Source: CAD feature listing. Evaluate the final solid. Frame: model axes, mm. A direction names the side the tool comes from. Round coordinates to 2 decimals unless told otherwise and drop trailing zeros. Loops run counter-clockwise (first coordinate to the right, second up) from the corner with the lowest first, then second, coordinate; pieces in that order, holes last. Notation, with made-up numbers: (32, 40) - (71, 40) arc R20 cw to (71, 55) - close; hole circle Ø6 at (-14, 39.25). An arc over 180 degrees is marked (long way). One line per question, with ' | ' between items. Start each with the question number.
1. Pin query (flat end, axial travel): pin 1 (1.7 mm diameter, centred on y = -2.5, z = 12, fed in from -X); pin 2 (2 mm diameter, centred on x = 39.5, y = -2, fed in from +Z); pin 3 (10 mm diameter, centred on x = 16, z = -22.5, fed in from +Y); pin 4 (0.5 mm diameter, centred on x = 10.5, y = -1.5, fed in from -Z). Return the tip coordinate at first contact, or that it passes through.
2. Access query for faces 1 (the flat face through (-24.002, -4.696, 13.889)), 2 (the flat face through (28.31, -3.131, 13.246)), 3 (the flat face through (20.5, -7.9, 38.2)). Directions: +Z, -Z, +X, -X, +Y, -Y. A direction counts if a zero-diameter tool reaches every point of the face in a straight line with its end or side. Return the directions, or none.
3. Ray query, line 1 (Z direction, x = -22, y = -3.5); line 2 (X direction, y = -8, z = 24); line 3 (Y direction, x = 4, z = -13). Return the intervals inside material, ascending.
4. Mould query, pull axis X, two halves, no side actions, for faces 4 (the flat face through (22.65, -3.13, 47.75)), 5 (the flat face through (30.569, -3, 13)), 6 (the flat face through (-12.87, -4.7, -18.37)). Classes: pulls with the +X half, pulls with the -X half, needs draft (parallel to the pull), parting line crosses it, or undercut.
5. Cut plane C-C (y = -2.5). State how many separate pieces and enclosed holes the cut face has, then the cut area to 3 significant figures.
6. Cut plane B-B (x = 44.5). Return loops of the section in (y, z) (3 decimals).
```python
from build123d import *

# Parameters (mm, degrees)
F1_DEPTH = 6.35
F3_DEPTH = 3.175


with BuildPart() as f1:
    # F0 (on Front) → F1 (new body)
    with BuildSketch(Plane.XZ):
        Polygon((36.4045640823, 1.9488933967), (69.6907226001, 26.065217087), (29.1461811696, 26.1190709712), (15.9708538221, 69.9924798862), (1.6629783111, 26.15557594), (-41.0424164863, 26.2123000095), (-6.4774139305, 1.2147947246), (-19.4446871391, -38.5147311336), (14.4759376997, -13.9387270281), (48.5830571498, -38.6050899867), align=None)
        with BuildLine():
            add(Edge.make_bspline(
                [(1.0703261445, 8.6234759039), (0.6811166374, 8.1998862237), (-0.0492998709, 8.1998862237)],
                knots=[0, 0, 0, 1, 1, 1], degree=2))
            add(Edge.make_bspline(
                [(-0.0492998709, 8.1998862237), (-0.4294278228, 8.1998862237), (-0.6486825118, 8.3088648857)],
                knots=[0, 0, 0, 1, 1, 1], degree=2))
            Line((-0.6486825118, 8.3088648857), (-0.6486825118, 8.8965712414))
            add(Edge.make_bspline(
                [(-0.6486825118, 8.8965712414), (-0.3606674766, 8.81613461), (-0.0492998709, 8.81613461)],
                knots=[0, 0, 0, 1, 1, 1], degree=2))
            add(Edge.make_bspline(
                [(-0.0492998709, 8.81613461), (0.3528832864, 8.81613461), (0.5617590552, 9.0593905519)],
                knots=[0, 0, 0, 1, 1, 1], degree=2))
            add(Edge.make_bspline(
                [(0.5617590552, 9.0593905519), (0.7706348241, 9.3026464938), (0.7706348241, 9.7606163472)],
                knots=[0, 0, 0, 1, 1, 1], degree=2))
            Line((0.7706348241, 9.7606163472), (0.7706348241, 15.6882771403))
            Line((0.7706348241, 15.6882771403), (1.4595356516, 15.6882771403))
            Line((1.4595356516, 15.6882771403), (1.4595356516, 9.8177004082))
            add(Edge.make_bspline(
                [(1.4595356516, 9.8177004082), (1.4595356516, 9.0470655842), (1.0703261445, 8.6234759039)],
                knots=[0, 0, 0, 1, 1, 1], degree=2))
        make_face(mode=Mode.SUBTRACT)
        with BuildLine():
            add(Edge.make_bspline(
                [(7.4598488861, 14.9708342823), (8.1772917442, 14.1599811425), (8.1772917442, 12.7328796164)],
                knots=[0, 0, 0, 1, 1, 1], degree=2))
            add(Edge.make_bspline(
                [(8.1772917442, 12.7328796164), (8.1772917442, 11.3096701855), (7.4572541561, 10.4942762681)],
                knots=[0, 0, 0, 1, 1, 1], degree=2))
            add(Edge.make_bspline(
                [(7.4572541561, 10.4942762681), (6.7372165679, 9.6788823507), (5.4567172896, 9.6788823507)],
                knots=[0, 0, 0, 1, 1, 1], degree=2))
            add(Edge.make_bspline(
                [(5.4567172896, 9.6788823507), (4.1476759807, 9.6788823507), (3.4360712652, 10.4800052528)],
                knots=[0, 0, 0, 1, 1, 1], degree=2))
            add(Edge.make_bspline(
                [(3.4360712652, 10.4800052528), (2.7244665497, 11.2811281549), (2.7244665497, 12.7406638066)],
                knots=[0, 0, 0, 1, 1, 1], degree=2))
            add(Edge.make_bspline(
                [(2.7244665497, 12.7406638066), (2.7244665497, 14.188523173), (3.4380173127, 14.9851052975)],
                knots=[0, 0, 0, 1, 1, 1], degree=2))
            add(Edge.make_bspline(
                [(3.4380173127, 14.9851052975), (4.1515680757, 15.781687422), (5.4645014797, 15.781687422)],
                knots=[0, 0, 0, 1, 1, 1], degree=2))
            add(Edge.make_bspline(
                [(5.4645014797, 15.781687422), (6.742406028, 15.781687422), (7.4598488861, 14.9708342823)],
                knots=[0, 0, 0, 1, 1, 1], degree=2))
        make_face(mode=Mode.SUBTRACT)
        with BuildLine():
            Line((11.4245963984, 12.2256098922), (10.1869101659, 12.2256098922))
            Line((10.1869101659, 12.2256098922), (10.1869101659, 9.7606163472))
            Line((10.1869101659, 9.7606163472), (9.4980093383, 9.7606163472))
            Line((9.4980093383, 9.7606163472), (9.4980093383, 15.6882771403))
            Line((9.4980093383, 15.6882771403), (11.1236077129, 15.6882771403))
            add(Edge.make_bspline(
                [(11.1236077129, 15.6882771403), (12.2146916979, 15.6882771403), (12.7355837549, 15.2705256027)],
                knots=[0, 0, 0, 1, 1, 1], degree=2))
            add(Edge.make_bspline(
                [(12.7355837549, 15.2705256027), (13.2564758119, 14.8527740651), (13.2564758119, 14.0133788948)],
                knots=[0, 0, 0, 1, 1, 1], degree=2))
            add(Edge.make_bspline(
                [(13.2564758119, 14.0133788948), (13.2564758119, 12.8379661833), (12.0641973551, 12.4241067408)],
                knots=[0, 0, 0, 1, 1, 1], degree=2))
            Line((12.0641973551, 12.4241067408), (13.6742273495, 9.7606163472))
            Line((13.6742273495, 9.7606163472), (12.8594821146, 9.7606163472))
            Line((12.8594821146, 9.7606163472), (11.4245963984, 12.2256098922))
        make_face(mode=Mode.SUBTRACT)
        with BuildLine():
            add(Edge.make_bspline(
                [(18.5957815668, 14.9221830939), (19.3618756133, 14.1560890474), (19.3618756133, 12.7808821223)],
                knots=[0, 0, 0, 1, 1, 1], degree=2))
            add(Edge.make_bspline(
                [(19.3618756133, 12.7808821223), (19.3618756133, 11.3135622805), (18.5652934887, 10.5370893139)],
                knots=[0, 0, 0, 1, 1, 1], degree=2))
            add(Edge.make_bspline(
                [(18.5652934887, 10.5370893139), (17.7687113642, 9.7606163472), (16.2728494919, 9.7606163472)],
                knots=[0, 0, 0, 1, 1, 1], degree=2))
            Line((16.2728494919, 9.7606163472), (14.6303853719, 9.7606163472))
            Line((14.6303853719, 9.7606163472), (14.6303853719, 15.6882771403))
            Line((14.6303853719, 15.6882771403), (16.4466964051, 15.6882771403))
            add(Edge.make_bspline(
                [(16.4466964051, 15.6882771403), (17.8296875203, 15.6882771403), (18.5957815668, 14.9221830939)],
                knots=[0, 0, 0, 1, 1, 1], degree=2))
        make_face(mode=Mode.SUBTRACT)
        Polygon((25.1234736834, 9.7606163472), (24.4099229204, 9.7606163472), (23.6717222219, 11.6456877266), (21.2962468635, 11.6456877266), (20.5671277202, 9.7606163472), (19.8691453375, 9.7606163472), (22.2121865703, 15.7129270758), (22.7921087358, 15.7129270758), align=None, mode=Mode.SUBTRACT)
        with BuildLine():
            Line((30.5685146877, 15.6882771403), (30.5685146877, 9.7606163472))
            Line((30.5685146877, 9.7606163472), (29.7823114834, 9.7606163472))
            Line((29.7823114834, 9.7606163472), (26.5427910193, 14.7347138479))
            Line((26.5427910193, 14.7347138479), (26.5103568937, 14.7347138479))
            add(Edge.make_bspline(
                [(26.5103568937, 14.7347138479), (26.5752251449, 13.858992457), (26.5752251449, 13.1298733137)],
                knots=[0, 0, 0, 1, 1, 1], degree=2))
            Line((26.5752251449, 13.1298733137), (26.5752251449, 9.7606163472))
            Line((26.5752251449, 9.7606163472), (25.9382189182, 9.7606163472))
            Line((25.9382189182, 9.7606163472), (25.9382189182, 15.6882771403))
            Line((25.9382189182, 15.6882771403), (26.7166379324, 15.6882771403))
            Line((26.7166379324, 15.6882771403), (29.9483742064, 10.7336401149))
            Line((29.9483742064, 10.7336401149), (29.980808332, 10.7336401149))
            add(Edge.make_bspline(
                [(29.980808332, 10.7336401149), (29.9730241418, 10.8426187769), (29.9444821113, 11.4368119578)],
                knots=[0, 0, 0, 1, 1, 1], degree=2))
            add(Edge.make_bspline(
                [(29.9444821113, 11.4368119578), (29.9159400808, 12.0310051386), (29.9237242709, 12.2865860483)],
                knots=[0, 0, 0, 1, 1, 1], degree=2))
            Line((29.9237242709, 12.2865860483), (29.9237242709, 15.6882771403))
            Line((29.9237242709, 15.6882771403), (30.5685146877, 15.6882771403))
        make_face(mode=Mode.SUBTRACT)
    extrude(amount=F1_DEPTH)

    # F2 (on face) → F3 (join)
    with BuildSketch(Plane.XZ.offset(6.35)):
        Polygon((36.4045640823, 1.9488933967), (69.4127031084, 25.8637877737), (28.9641653483, 25.9175141396), (15.8445339726, 69.6054572911), (1.6629783111, 26.15557594), (1.5467987544, 26.1557302572), (1.4809624898, 25.9540191084), (-40.7628684516, 26.0101300989), (-6.4774139305, 1.2147947246), (-19.4446871391, -38.5147311336), (14.4759376997, -13.9387270281), (48.2732234246, -38.3810173811), (36.222548261, 1.7473365651), (36.421750894, 1.891661876), align=None)
        Polygon((55.4314800111, 21.3103554065), (30.9093811696, 3.5437250843), (40.1384522175, -27.1887794914), (14.2914917683, -8.4961863292), (-10.9143527112, -26.7582006747), (-1.2785905938, 2.7641402252), (-27.0746829363, 21.4199454322), (4.7966385236, 21.3776118802), (15.6072232815, 54.4994101005), (25.5620899488, 21.3500298636), align=None, mode=Mode.SUBTRACT)
    extrude(amount=F3_DEPTH)


solid = f1.part
```
Answers follow:
1) pin 1: stops at x = -22.57 | pin 2: stops at z = 26.11 | pin 3: passes through | pin 4: stops at z = -17
2) face 1: -X, +Y, -Y | face 2: +Y, -Y | face 3: -Y
3) line 1: z = 12.44 to 26.19 | line 2: x = -37.98 to 5.65, 24.77 to 66.84 | line 3: y = -6.35 to 0
4) face 4: pulls with the +X half | face 5: undercut | face 6: pulls with the -X half
5) separate pieces: 1 | enclosed holes: 6 | area: 3,780 mm2
6) outline: (-9.525, -35.652) - (0, -35.652) - (0, -25.009) - (-6.35, -25.009) - (-6.35, -25.816) - (-9.525, -25.816) - close; (-9.525, 7.814) - (0, 7.814) - (0, 26.099) - (-6.35, 26.099) - (-6.35, 25.897) - (-9.525, 25.897) - (-9.525, 21.325) - (-6.35, 21.325) - (-6.35, 13.39) - (-9.525, 13.39) - close
